from build123d import *

# Parameters (mm, degrees)
F0_W     = 239.15
F0_H     = 87.15
F0_W_2   = 234
F0_H_2   = 82
F0_W_3   = 233
F0_H_3   = 81
F0_W_4   = 226.65
F0_H_4   = 74.65
F1_DEPTH = 12.525
F2_W     = 234
F2_H     = 82
F2_W_2   = 233
F2_H_2   = 81
F2_W_3   = 226.65
F2_H_3   = 74.65
F3_DEPTH = 1.5
F4_W     = 234
F4_H     = 82
F4_W_2   = 233
F4_H_2   = 81
F4_W_3   = 226.65
F4_H_3   = 74.65
F5_DEPTH = 1.5
F6_W     = 16
F6_H     = 9
F7_DEPTH = 10
F8_R     = 2


# Not quite as in the source:
# - a pattern or mirror of a feature is missing from the dataset's text; its kind, count and spacing are read off the source's solid


with BuildPart() as f1:
    # F0 (on Top) → F1 (new body)
    with BuildSketch(Plane.XY):
        Rectangle(F0_W, F0_H)
        Rectangle(F0_W_2, F0_H_2, mode=Mode.SUBTRACT)
        Rectangle(F0_W_2, F0_H_2)
        Rectangle(F0_W_3, F0_H_3, mode=Mode.SUBTRACT)
        Rectangle(F0_W_3, F0_H_3)
        Rectangle(F0_W_4, F0_H_4, mode=Mode.SUBTRACT)
    extrude(amount=F1_DEPTH)

    # F2 (on face) → F3 (cut)
    with BuildSketch(Plane.XY.offset(12.525)):
        Rectangle(F2_W, F2_H)
        Rectangle(F2_W_2, F2_H_2, mode=Mode.SUBTRACT)
        Rectangle(F2_W_2, F2_H_2)
        Rectangle(F2_W_3, F2_H_3, mode=Mode.SUBTRACT)
    f3 = extrude(amount=-F3_DEPTH, mode=Mode.SUBTRACT)

    # F3_copies: F3 across plane
    add(f3.mirror(Plane(origin=(0, 0, 6.2625), x_dir=(-1, 0, 0), z_dir=(0, 0, -1))), mode=Mode.SUBTRACT)

    # F4 (on face) → F5 (cut)
    with BuildSketch(Plane.XY):
        Rectangle(F4_W, F4_H)
        Rectangle(F4_W_2, F4_H_2, mode=Mode.SUBTRACT)
        Rectangle(F4_W_2, F4_H_2)
        Rectangle(F4_W_3, F4_H_3, mode=Mode.SUBTRACT)
    extrude(amount=-F5_DEPTH, mode=Mode.SUBTRACT)

    # F6 (on face) → F7 (cut)
    with BuildSketch(Plane.XZ.offset(43.575)):
        with Locations((-79.875, 8.5)):
            Rectangle(F6_W, F6_H)
    extrude(amount=-F7_DEPTH, mode=Mode.SUBTRACT)

    # F8
    f8_edges = [f1.edges().sort_by_distance(p)[0] for p in [
        (-71.875, -40.45, 4),
        (-87.875, -40.45, 4),
    ]]
    fillet(f8_edges, radius=F8_R)


solid = f1.part
The model under review builds one solid part; all positions refer to its coordinate system, in mm. A direction names the side the tool comes from. Give positions to 0.01 mm unless a question says otherwise; leave off trailing zeros. Order: outer loops, then holes, each group sorted by start corner. A loop starts at its lowest first (then second) coordinate and runs counter-clockwise, first axis right, second up. Notation, with made-up numbers: M 25,22.5 L 64,22.5 A20 cw 64,29.5 Z; hole C -38.5,7.25 d1. An arc over 180 degrees is marked long. Answer in a Markdown table with one row per item. Add a question column.
1. Add section A-A on x = 78. State the section outline as (y, z) points (3 decimals).
2. To check wall thickness, follow line 1 along Y through (x, z) = (56, 9.5) (3 decimals); line 2 along X through (y, z) = (15, 11.5) (3 decimals); line 3 along Y through (x, z) = (2.5, 1) (3 decimals). State the ranges of each line that lie inside material, in increasing order.
3. Add section B-B on y = 14.5. State the section outline as (x, z) points (3 decimals), plus the area to 3 significant figures.
4. Mouldability with a two-part tool opening along Y and no side actions: class faces 1 (the flat face through (-2, -43.575, 6)), 2 (the flat face through (-1, 42, 12.525)), 3 (the flat face through (-1, 40, 1.5)), 4 (the flat face through (-1, 40, 11.025)) as released by +Y, released by -Y, zero draft, split by the parting line, or undercut.
5. Add section C-C on z = 8.5. State the section outline as (x, y) points (3 decimals).
6. Machinability: for faces 5 (the flat face through (-71.875, -40, 9)), 6 (the flat face through (-2, -37.325, 6)), 7 (the flat face through (-119.575, -1, 6)), which of the approach directions +Z, -Z, +X, -X, +Y, -Y give a long, thin tool a straight path to every point of the face, cutting with its end or side? Answer none if there is none.
7. For pin 1 Ø24.5 at (x, y) = (20, -18.5) entering from -Z; pin 2 Ø1.9 at (x, y) = (-81, -41) entering from +Z, all flat-tipped, find the tip position at first contact; note any pin that passes through.
The answers:
| question | item | result |
|---|---|---|
| 1 | outline | M -43.575,0 L -41,0 L -41,1.5 L -37.325,1.5 L -37.325,11.025 L -41,11.025 L -41,12.525 L -43.575,12.525 Z; M 37.325,1.5 L 41,1.5 L 41,0 L 43.575,0 L 43.575,12.525 L 41,12.525 L 41,11.025 L 37.325,11.025 Z |
| 2 | line 1 | -43.575 to -37.325, 37.325 to 43.575 |
| 2 | line 2 | -119.575 to -117, 117 to 119.575 |
| 2 | line 3 | -43.575 to -41, 41 to 43.575 |
| 3 | outline | M -119.575,0 L -117,0 L -117,1.5 L -113.325,1.5 L -113.325,11.025 L -117,11.025 L -117,12.525 L -119.575,12.525 Z; M 113.325,1.5 L 117,1.5 L 117,0 L 119.575,0 L 119.575,12.525 L 117,12.525 L 117,11.025 L 113.325,11.025 Z |
| 3 | area | 135 mm2 |
| 4 | face 1 | released by -Y |
| 4 | face 2 | zero draft |
| 4 | face 3 | undercut |
| 4 | face 4 | undercut |
| 5 | outline | M -119.575,-43.575 L -87.875,-43.575 L -87.875,-37.325 L -113.325,-37.325 L -113.325,37.325 L 113.325,37.325 L 113.325,-37.325 L -71.875,-37.325 L -71.875,-43.575 L 119.575,-43.575 L 119.575,43.575 L -119.575,43.575 Z |
| 6 | face 5 | +Z, -Y |
| 6 | face 6 | +Z, -Z |
| 6 | face 7 | +Z, -Z, -X, +Y, -Y |
| 7 | pin 1 | through |
| 7 | pin 2 | z = 4 |
